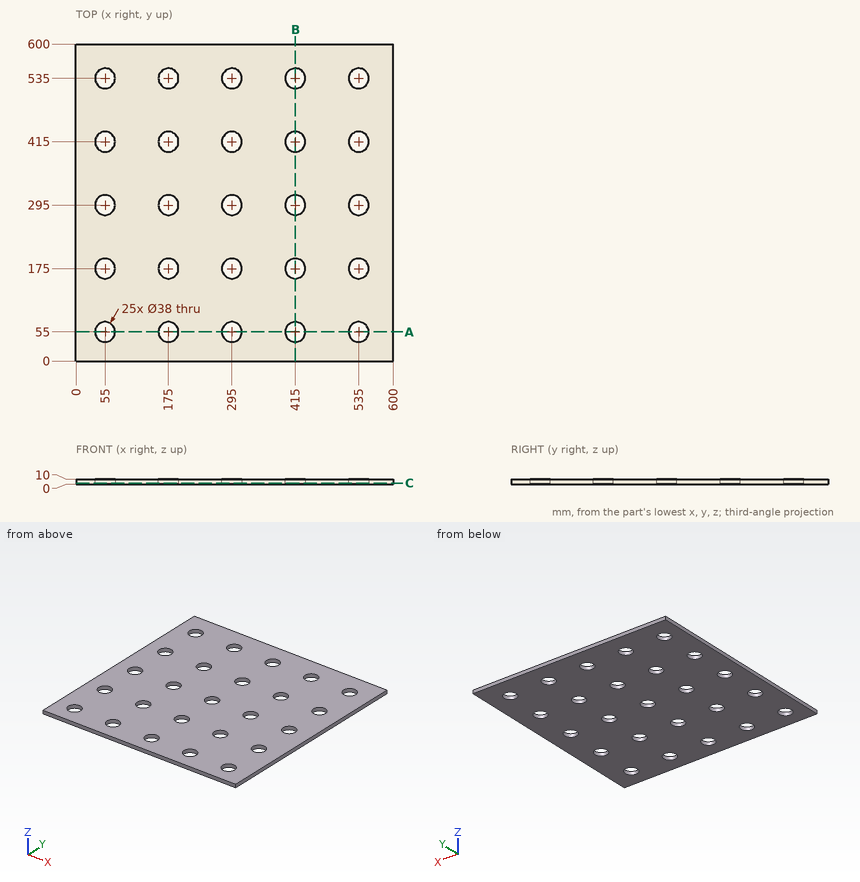
Can you work these out from the drawing? Everything is in mm from the part's minimum corner. Give positions to 0.01 mm unless a question says otherwise; leave off trailing zeros. Order: outer loops, then holes, each group sorted by start corner. A loop starts at its lowest first (then second) coordinate and runs counter-clockwise, first axis right, second up. Notation, with made-up numbers: M 81.25,27.5 L 106.25,27.5 A17 cw 106.25,56.5 Z; hole C -30.5,30 d7. An arc over 180 degrees is marked long. Use a Markdown table: item, result. Add a question column.
1. Suppose I cut it at C-C (z = 2). Give the number of separate pieces and of enclosed holes in the cut face, and give its area (3 significant figures).
2. I need wall thicknesses on probe 1 along Y at (x, z) = (295, 6.5); probe 2 along Y at (x, z) = (65.5, 5). Which ranges of each line are inside material? Lowest first, please. Write a range as from..to.
3. For pin 1 Ø3 at (x, y) = (290.5, 326) entering from -Z; pin 2 Ø23 at (x, y) = (175, 295) entering from -Z (3 decimals), each with a flat end and sliding along its axis, tell me the tip position at first contact or that it passes through.
4. Suppose I cut it at A-A (y = 55). List the corners of the cut face in (x, z) for me, and give its area (3 significant figures).
Results list:
| question | item | result |
|---|---|---|
| 1 | separate pieces | 1 |
| 1 | enclosed holes | 25 |
| 1 | area | 332,000 mm² |
| 2 | probe 1 | y = 0..36, 74..156, 194..276, 314..396, 434..516, 554..600 |
| 2 | probe 2 | y = 0..39.16, 70.84..159.16, 190.84..279.16, 310.84..399.16, 430.84..519.16, 550.84..600 |
| 3 | pin 1 | stops at z = 0 |
| 3 | pin 2 | passes through |
| 4 | outline | M 0,0 L 36,0 L 36,10 L 0,10 Z; M 74,0 L 156,0 L 156,10 L 74,10 Z; M 194,0 L 276,0 L 276,10 L 194,10 Z; M 314,0 L 396,0 L 396,10 L 314,10 Z; M 434,0 L 516,0 L 516,10 L 434,10 Z; M 554,0 L 600,0 L 600,10 L 554,10 Z |
| 4 | area | 4,100 mm² |
